from build123d import *

# Parameters (mm, degrees)
SKETCH1_R           = 1.5
SKETCH1_R_2         = 1.905
BOSS_EXTRUDE1_DEPTH = 2.54


with BuildPart() as part:
    # Sketch1 → Boss-Extrude1 (new body)
    with BuildSketch(Plane.XY):
        Polygon((-7.213493432, 12.767883374), (-14.66405807, 0.136873125), (-7.450564639, -12.631010249), (7.213493432, -12.767883374), (14.66405807, -0.136873125), (7.450564639, 12.631010249), align=None)
        with Locations((-8.509, 0.079422314)):
            Circle(SKETCH1_R, mode=Mode.SUBTRACT)
        with Locations((8.509, -0.079422314)):
            Circle(SKETCH1_R, mode=Mode.SUBTRACT)
        Circle(SKETCH1_R_2, mode=Mode.SUBTRACT)
    extrude(amount=BOSS_EXTRUDE1_DEPTH)


solid = part.part
Verification items for the finished model (mm, model axes). Give positions to 0.01 mm unless a question says otherwise; leave off trailing zeros. Loops run counter-clockwise (first coordinate to the right, second up) from the corner with the lowest first, then second, coordinate; pieces in that order, holes last. Notation, with made-up numbers: (-19, -25) - (0, -25) arc R21 cw to (0, -4) - close; hole circle Ø4 at (38.5, 13). An arc over 180 degrees is marked (long way). Write item = value, one per line. Start each with the question number.
Q1. Mould release check, pull along X, two halves, no side actions. Record for faces 1 (the face through (11.108, 6.158, 1.252)), 2 (the face through (-8.834, -1.385, 1.252)), 3 (the face through (-11.108, -6.158, 1.252)), 4 (the face through (9.895, -0.654, 1.252)): released by +X, released by -X, zero draft, split by the parting line, or undercut.
Q2. Depth check by flat-ended pin: P1, Ø1, axis at x = -11, z = 1, coming from the +Y side. Enter the tip coordinate at first touch or a pass-through.
Q3. Cross-section at D-D, the plane x = 0. Enter the section's corners in (y, z) (3 decimals), and give its area (3 significant figures).
Q4. Cross-section at C-C, the plane y = -2.5. Enter the section's corners in (x, z), and give its area (3 significant figures).
Q5. Cross-section at A-A, the plane x = 8. Enter the section's corners in (y, z), and give its area (3 significant figures).
Q6. Cross-section at B-B, the plane z = 0.4. Enter the section's corners in (x, y) (1 decimal), and give its area (3 significant figures).
Q7. Thickness scan on line 1 (Y direction, x = 0, z = 1.8) (3 decimals); line 2 (Y direction, x = -1.75, z = 1.75); line 3 (X direction, y = 1.25, z = 2.05). Record the ranges inside material, lowest first.
Answer key:
q1.face_1 = released by +X
q1.face_2 = undercut
q1.face_3 = released by -X
q1.face_4 = undercut
q2.P1 = 7.2
q3.outline = (-12.701, 0) - (-1.905, 0) - (-1.905, 2.54) - (-12.701, 2.54) - close; (1.905, 0) - (12.701, 0) - (12.701, 2.54) - (1.905, 2.54) - close
q3.area = 54.8 mm^2
q4.outline = (-13.17, 0) - (13.27, 0) - (13.27, 2.54) - (-13.17, 2.54) - close
q4.area = 67.2 mm^2
q5.outline = (-11.43, 0) - (-1.49, 0) - (-1.49, 2.54) - (-11.43, 2.54) - close; (1.33, 0) - (11.66, 0) - (11.66, 2.54) - (1.33, 2.54) - close
q5.area = 51.5 mm^2
q6.outline = (-14.7, 0.1) - (-7.5, -12.6) - (7.2, -12.8) - (14.7, -0.1) - (7.5, 12.6) - (-7.2, 12.8) - close; hole circle Ø3 at (-8.5, 0.1); hole circle Ø3.8 at (0, 0); hole circle Ø3 at (8.5, -0.1)
q6.area = 533 mm^2
q7.line_1 = -12.701 to -1.905, 1.905 to 12.701
q7.line_2 = -12.68 to -0.75, 0.75 to 12.72
q7.line_3 = -14.01 to -9.45, -7.57 to -1.44, 1.44 to 7.81, 9.2 to 13.88
